For this review, take the finished solid that the model builds, in its own axes (mm). Coordinates: 2 decimals unless noted, no trailing zeros. Write each loop counter-clockwise with the first axis right and the second up, starting at its lowest first coordinate (ties: lowest second). Pieces come first, ordered by that corner, then holes. Notation, with made-up numbers: (77, -6) - (86, -6) arc R17 ccw to (86, 4) - close; hole circle Ø2 at (30, -14.5). An arc over 180 degrees is marked (long way). Use one line per item in the form item = value. Start each with the question number.
1) We need section B-B (z = 1.85). Give the boundary of the cut face in (x, y), plus the area to 3 significant figures.
2) We need section A-A (x = 0). Give the boundary of the cut face in (y, z).
3) Insertion check: P1, Ø1.5, axis at x = -2.5, z = 1, coming from the +Y side; P2, Ø3, axis at x = -3, y = 65, coming from the -Z side. Each pin has a flat end and moves straight along its axis. Give the tip position at first contact, or say it passes through.
4) For L1, parallel to Y at x = 0, z = 1; L2, parallel to Y at x = 0.25, z = 1.5; L3, parallel to Y at x = 2.5, z = 2.8, list the stretches that pass through material, from the lowest coordinate up. Write a range as from..to.
5) Mouldability with a two-part tool opening along X and no side actions: class faces 1 (the cylindrical face through (-0.43, 111.71, 1.48)), 2 (the flat face through (-4, 61, 1)), 3 (the flat face through (0, 61, 0)), 4 (the cylindrical face through (-0.088, 113.756, 1.479)) as pulls with the +X half, pulls with the -X half, needs draft (parallel to the pull), parting line crosses it, or undercut.
Autodesk Inventor part; units mm, degrees
ref_plane "YZ Plane" through (0, 0, 0) normal (1, 0, 0) x (0, 1, 0)
ref_plane "XZ Plane" through (0, 0, 0) normal (0, 1, 0) x (-1, 0, 0)
ref_plane "XY Plane" through (0, 0, 0) normal (0, 0, 1) x (1, 0, 0)
ref_plane "Work Plane1" through (0, 0, 0) normal (0, 0, 1) x (1, 0, 0)
sketch "Sketch1" plane through (0, 0, 0) normal (0, 0, 1) x (1, 0, 0)
  line L0 (-4.7216, 11.5478) -> (-13.9385, -14.9025)
  line L1 (-13.9385, -14.9025) -> (13.9385, -14.9025)
  line L2 (13.9385, -14.9025) -> (4.7216, 11.5478)
  arc A0 (4.7216, 11.5478) -> (-4.7216, 11.5478) centre (0, 9.9025) ccw
  circle A1 centre (0, 9.9025) radius 2
  line L3 (2, 139.4798) -> (-2, 139.4798)
  line L4 (4.7216, 108.1118) -> (13.9385, 134.5621)
  line L5 (13.9385, 134.5621) -> (-13.9385, 134.5621)
  line L6 (-13.9385, 134.5621) -> (-4.7216, 108.1118)
  arc A2 (-4.7216, 108.1118) -> (4.7216, 108.1118) centre (0, 109.7571) ccw
  circle A3 centre (0, 109.7571) radius 2
  line L7 (0, 9.9025) -> (0, 109.7571) construction
  line L8 (4, 9.9025) -> (4, 109.7571)
  line L9 (-4, 109.7571) -> (-4, 9.9025)
  arc A4 (-4, 9.9025) -> (4, 9.9025) centre (0, 9.9025) ccw
  arc A5 (4, 109.7571) -> (-4, 109.7571) centre (0, 109.7571) ccw
  point P0 (0, 0)
  point P1 (0, 59.8298)
  dimension "d0" = 8
extrude "Extrusion1" add sketch "Sketch1" along normal blind 3 contours L9 A2 L8 A0 | A0 L8 A4 L9 | L9 A5 L8 A2
properties part number "horizontal truss top"
Determined:
q1.outline = (-4, 9.9) arc R4 ccw to (4, 9.9) - (4, 109.76) arc R4 ccw to (-4, 109.76) - close; hole circle Ø4 at (0, 9.9); hole circle Ø4 at (0, 109.76)
q1.area = 824 mm²
q2.outline = (5.9, 0) - (7.9, 0) - (7.9, 3) - (5.9, 3) - close; (11.9, 0) - (107.76, 0) - (107.76, 3) - (11.9, 3) - close; (111.76, 0) - (113.76, 0) - (113.76, 3) - (111.76, 3) - close
q3.P1 = 113.35
q3.P2 = 0
q4.L1 = 5.9..7.9, 11.9..107.76, 111.76..113.76
q4.L2 = 5.91..7.92, 11.89..107.77, 111.74..113.75
q4.L3 = 6.78..112.88
q5.face_1 = undercut
q5.face_2 = pulls with the -X half
q5.face_3 = needs draft
q5.face_4 = parting line crosses it
